Input: part model. Units: mm. Frame: model coordinates. Face numbers are marked on the shaded views. A direction names the side the tool comes from. Give positions to 0.01 mm unless a question says otherwise; leave off trailing zeros. Write each loop counter-clockwise with the first axis right and the second up, starting at its lowest first coordinate (ties: lowest second). Pieces come first, ordered by that corner, then holes. Notation, with made-up numbers: (46.25, 78.25) -> (50.25, 78.25) arc R22 cw to (50.25, 107.25) -> close; hole circle Ø9 at (6, 55.5). An arc over 180 degrees is marked (long way). Return JSON: item names as keys, results as strings. Group by question number.
Item 1: Section B-B, the plane z = 5. Return loops of the section in (x, y).
Item 2: Pin query (flat end, axial travel): P1, Ø0.7, axis at y = 4, z = -4.5, coming from the +X side; P2, Ø6, axis at x = 20.5, y = 5, coming from the -Z side; P3, Ø10, axis at x = 19, y = 15, coming from the -Z side; P4, Ø4, axis at x = 35.5, z = -8, coming from the -Y side. Return the tip coordinate at first contact, or that it passes through.
Item 3: Section D-D, the plane x = 20. Return loops of the section in (y, z), then the cut area to 3 significant figures.
Item 4: Mould query, pull axis Y, two halves, no side actions, for the marked faces 4, 5, 6 and 7. Classes: released by +Y, released by -Y, zero draft, split by the parting line, or undercut.
Item 5: Set-up query: the marked faces 1, 2 and 3. Return all of +Z, -Z, +X, -X, +Y, -Y with unobstructed straight access to the full face (end or side cutting, diameter ignored); none if empty.
Item 6: Section A-A, the plane y = 13.5. Return loops of the section in (x, z), then the cut area to 3 significant figures.
Item 7: Line query: line 1 (X direction, y = 17.5, z = 8); line 2 (Y direction, x = 29, z = 15); line 3 (X direction, y = 2.05, z = 25.2). Output: solid intervals per line, ascending. Write a range as [from, to].
Item 8: Section C-C, the plane x = 14. Return loops of the section in (y, z).
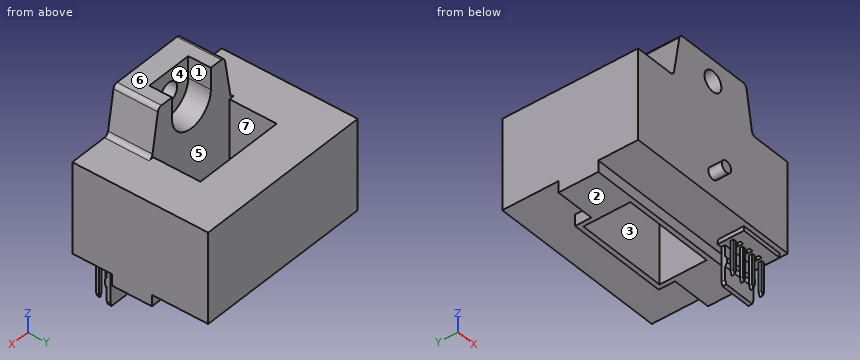
from build123d import *

# Parameters (mm, degrees)
SKETCH1_W                   = 40
SKETCH1_H                   = 30
SKETCH1_W_2                 = 20.4
SKETCH1_H_2                 = 10.4
BOSS_EXTRUDE1_DEPTH         = 20
BOSS_EXTRUDE2_DEPTH         = 9.8
CUT_EXTRUDE1_DEPTH          = 5
SKETCH4_R                   = 2.25
CUT_EXTRUDE2_DEPTH          = 56.991427915
SKETCH5_W                   = 8.8
SKETCH5_H                   = 8.8
SKETCH5_W_2                 = 20.4
SKETCH5_H_2                 = 10.4
BOSS_EXTRUDE3_DEPTH         = 2.5
SKETCH7_R                   = 1.25
BOSS_EXTRUDE4_DEPTH         = 3
BODY_MOVE_COPY6_START       = 1
BODY_MOVE_COPY6_DEPTH       = 4.9
BODY_MOVE_COPY6_START_2     = 5.95
BODY_MOVE_COPY6_2_DEPTH     = 0.85
BODY_MOVE_COPY6_START_3     = 3.8825
BODY_MOVE_COPY6_3_DEPTH     = 0.635
BODY_MOVE_COPY6_4_OUTLINE_W = 0.75
BODY_MOVE_COPY6_4_OUTLINE_H = 1
BODY_MOVE_COPY6_4_DEPTH     = 2.35
BODY_MOVE_COPY6_START_4     = 4.6
BODY_MOVE_COPY6_5_OUTLINE_W = 0.75
BODY_MOVE_COPY6_5_OUTLINE_H = 1
BODY_MOVE_COPY6_5_DEPTH     = 1.35
BODY_MOVE_COPY6_START_5     = 30.5
BODY_MOVE_COPY6_6_DEPTH     = 7.5
BODY_MOVE_COPY6_START_6     = 29.5
BODY_MOVE_COPY6_7_DEPTH     = 9.5


with BuildPart() as part:
    # Sketch1 → Boss-Extrude1 (new body)
    with BuildSketch(Plane.XY):
        with Locations((20, 15)):
            Rectangle(SKETCH1_W, SKETCH1_H)
        with Locations((20, 15)):
            Rectangle(SKETCH1_W_2, SKETCH1_H_2, mode=Mode.SUBTRACT)
    extrude(amount=BOSS_EXTRUDE1_DEPTH)

    # Sketch2 → Boss-Extrude2 (add)
    with BuildSketch(Plane.XZ):
        with BuildLine():
            Line((8.6, 20), (31.4, 20))
            ThreePointArc((31.4, 20), (30.755366169, 20.23550851), (30.414365834, 20.831105526))
            Line((30.414365834, 20.831105526), (28.985634166, 29.168894474))
            ThreePointArc((28.985634166, 29.168894474), (28.644633831, 29.76449149), (28, 30))
            Line((28, 30), (12, 30))
            ThreePointArc((12, 30), (11.355366169, 29.76449149), (11.014365834, 29.168894474))
            Line((11.014365834, 29.168894474), (9.585634166, 20.831105526))
            ThreePointArc((9.585634166, 20.831105526), (9.244633831, 20.23550851), (8.6, 20))
        make_face()
    extrude(amount=-BOSS_EXTRUDE2_DEPTH)

    # Sketch3 → Cut-Extrude1 (cut)
    with BuildSketch(Plane(origin=(0, 9.8, 0), x_dir=(1, 0, 0), z_dir=(0, 1, 0))):
        with BuildLine():
            Line((25.2, -25.2), (25.2, -30))
            Line((25.2, -30), (14.8, -30))
            Line((14.8, -30), (14.8, -25.2))
            ThreePointArc((14.8, -25.2), (20, -20), (25.2, -25.2))
        make_face()
    extrude(amount=-CUT_EXTRUDE1_DEPTH, mode=Mode.SUBTRACT)

    # Sketch4 → Cut-Extrude2 (cut, through all)
    with BuildSketch(Plane(origin=(0, 4.8, 0), x_dir=(1, 0, 0), z_dir=(0, 1, 0))):
        with Locations(Location((20, -25.2, 0), (0, 0, 270))):
            Circle(SKETCH4_R)
    extrude(amount=-CUT_EXTRUDE2_DEPTH, mode=Mode.SUBTRACT)

    # Sketch5 → Boss-Extrude3 (add)
    # profile 1 of 3: a face of its own
    with BuildSketch(Plane(origin=(0, 0, 0), x_dir=(-1, 0, 0), z_dir=(0, 0, -1))):
        with Locations((-4.4, 13.2)):
            Rectangle(SKETCH5_W, SKETCH5_H)
    # profile 2 of 3: a face of its own
    with BuildSketch(Plane(origin=(0, 0, 0), x_dir=(-1, 0, 0), z_dir=(0, 0, -1))):
        Polygon((-31.2, 8.8), (-8.8, 8.8), (-8.8, 17.6), (-8.8, 21.2), (-31.2, 21.2), (-31.2, 17.6), align=None)
        with Locations((-20, 15)):
            Rectangle(SKETCH5_W_2, SKETCH5_H_2, mode=Mode.SUBTRACT)
    # profile 3 of 3: a face of its own
    with BuildSketch(Plane(origin=(0, 0, 0), x_dir=(-1, 0, 0), z_dir=(0, 0, -1))):
        with Locations((-35.6, 13.2)):
            Rectangle(SKETCH5_W, SKETCH5_H)
    extrude(amount=BOSS_EXTRUDE3_DEPTH)

    # Sketch7 → Boss-Extrude4 (add)
    with BuildSketch(Plane.XZ):
        with Locations(Location((20, 5, 0), (0, 0, 90))):
            Circle(SKETCH7_R)
    extrude(amount=BOSS_EXTRUDE4_DEPTH)


with BuildPart() as body_2:
    # Body-Move/Copy6: read off the stored shape, not the designer's step
    # Body-Move/Copy6 outline → Body-Move/Copy6 (new body)
    with BuildSketch(Plane(origin=(0, 0, 0), x_dir=(1, 0, 0), z_dir=(0, 1, 0)).offset(BODY_MOVE_COPY6_START)):
        Polygon((34.75, -1.3), (36.25, -1.3), (36.25, -2.3), (37.25, -2.3), (37.25, -1.3), (38.75, -1.3), (38.75, -2.3), (39, -2.3), (39, 1), (37.125, 1), (37.125, 0), (36.375, 0), (36.375, 1), (34.625, 1), (34.625, 0), (33.875, 0), (33.875, 1), (32.125, 1), (32.125, 0), (31.375, 0), (31.375, 1), (29.5, 1), (29.5, -2.3), (29.75, -2.3), (29.75, -1.3), (31.25, -1.3), (31.25, -2.3), (32.25, -2.3), (32.25, -1.3), (33.75, -1.3), (33.75, -2.3), (34.75, -2.3), align=None)
    extrude(amount=BODY_MOVE_COPY6_DEPTH)

    # Body-Move_Copy6 2 outline → Body-Move_Copy6 2 (add)
    with BuildSketch(Plane(origin=(0, 0, 0), x_dir=(1, 0, 0), z_dir=(0, 1, 0)).offset(BODY_MOVE_COPY6_START_2)):
        Polygon((38, 1), (38, 8.6), (37.708823813, 9.4), (30.791176187, 9.4), (30.5, 8.6), (30.5, 1), align=None)
    extrude(amount=BODY_MOVE_COPY6_2_DEPTH)

    # Body-Move_Copy6 3 outline → Body-Move_Copy6 3 (add)
    with BuildSketch(Plane(origin=(0, 0, 0), x_dir=(1, 0, 0), z_dir=(0, 1, 0)).offset(BODY_MOVE_COPY6_START_3)):
        Polygon((35.1825, -4.827675919), (35.5, -5.7), (35.8175, -4.827675919), (35.8175, -1.3), (35.1825, -1.3), align=None)
        Polygon((38.3175, -1.3), (37.6825, -1.3), (37.6825, -4.827675919), (38, -5.7), (38.3175, -4.827675919), align=None)
        Polygon((33.3175, -4.827675919), (33.3175, -1.3), (32.6825, -1.3), (32.6825, -4.827675919), (33, -5.7), align=None)
        Polygon((38.3175, 1), (38.3175, 7.627675919), (38, 8.5), (37.6825, 7.627675919), (37.6825, 1), align=None)
        Polygon((30.8175, -4.827675919), (30.8175, -1.3), (30.1825, -1.3), (30.1825, -4.827675919), (30.5, -5.7), align=None)
        Polygon((35.1825, 1), (35.8175, 1), (35.8175, 7.627675919), (35.5, 8.5), (35.1825, 7.627675919), align=None)
        Polygon((30.1825, 7.627675919), (30.1825, 1), (30.8175, 1), (30.8175, 7.627675919), (30.5, 8.5), align=None)
        Polygon((32.6825, 1), (33.3175, 1), (33.3175, 7.627675919), (33, 8.5), (32.6825, 7.627675919), align=None)
    extrude(amount=BODY_MOVE_COPY6_3_DEPTH)

    # Body-Move_Copy6 4 outline → Body-Move_Copy6 4 (add)
    with BuildSketch(Plane(origin=(0, 0, 0), x_dir=(1, 0, 0), z_dir=(0, 1, 0)).offset(BODY_MOVE_COPY6_START)):
        with Locations((36.75, 0.5)):
            Rectangle(BODY_MOVE_COPY6_4_OUTLINE_W, BODY_MOVE_COPY6_4_OUTLINE_H)
        with Locations((34.25, 0.5)):
            Rectangle(BODY_MOVE_COPY6_4_OUTLINE_W, BODY_MOVE_COPY6_4_OUTLINE_H)
        with Locations((31.75, 0.5)):
            Rectangle(BODY_MOVE_COPY6_4_OUTLINE_W, BODY_MOVE_COPY6_4_OUTLINE_H)
    extrude(amount=BODY_MOVE_COPY6_4_DEPTH)

    # Body-Move_Copy6 5 outline → Body-Move_Copy6 5 (add)
    with BuildSketch(Plane(origin=(0, 0, 0), x_dir=(1, 0, 0), z_dir=(0, 1, 0)).offset(BODY_MOVE_COPY6_START_4)):
        with Locations((36.75, 0.5)):
            Rectangle(BODY_MOVE_COPY6_5_OUTLINE_W, BODY_MOVE_COPY6_5_OUTLINE_H)
        with Locations((34.25, 0.5)):
            Rectangle(BODY_MOVE_COPY6_5_OUTLINE_W, BODY_MOVE_COPY6_5_OUTLINE_H)
        with Locations((31.75, 0.5)):
            Rectangle(BODY_MOVE_COPY6_5_OUTLINE_W, BODY_MOVE_COPY6_5_OUTLINE_H)
    extrude(amount=BODY_MOVE_COPY6_5_DEPTH)

    # Body-Move_Copy6 6 outline → Body-Move_Copy6 6 (add)
    with BuildSketch(Plane.YZ.offset(BODY_MOVE_COPY6_START_5)):
        Polygon((5.95, -3.5), (5.55, -3.976701437), (5.55, -4.976701437), (5.95, -5.66952176), align=None)
        with BuildLine():
            Line((5.9, -1), (6.8, -1))
            Line((6.8, -1), (6.8, -0.6))
            ThreePointArc((6.8, -0.6), (6.536396103, 0.036396103), (5.9, 0.3))
            Line((5.9, 0.3), (5.9, -1))
        make_face()
    extrude(amount=BODY_MOVE_COPY6_6_DEPTH)

    # Body-Move_Copy6 7 outline → Body-Move_Copy6 7 (add)
    with BuildSketch(Plane.YZ.offset(BODY_MOVE_COPY6_START_6)):
        with BuildLine():
            Line((5.9, -1), (6.8, -1))
            Line((6.8, -1), (6.8, -0.6))
            ThreePointArc((6.8, -0.6), (6.536396103, 0.036396103), (5.9, 0.3))
            Line((5.9, 0.3), (5.9, -1))
        make_face()
    extrude(amount=BODY_MOVE_COPY6_7_DEPTH)


with BuildPart() as part_1:
    add(part.part)

    # Intersect3: read off the stored shape, not the designer's step
    # Intersect3: union body 2
    add(body_2.part)


solid = part_1.part
Answer below:
{
 "1": {"outline": "(0, 0) -> (18.75, 0) -> (18.75, -3) -> (21.25, -3) -> (21.25, 0) -> (40, 0) -> (40, 30) -> (0, 30) -> close; hole (9.8, 9.8) -> (30.2, 9.8) -> (30.2, 20.2) -> (9.8, 20.2) -> close"},
 "2": {"P1": "stops at x = 38.32", "P2": "stops at z = 0", "P3": "passes through", "P4": "stops at y = 3.88"},
 "3": {"outline": "(-3, 3.75) -> (0, 3.75) -> (0, 0) -> (8.8, 0) -> (8.8, -2.5) -> (9.8, -2.5) -> (9.8, 20) -> (4.8, 20) -> (4.8, 22.95) -> (0, 22.95) -> (0, 6.25) -> (-3, 6.25) -> close; (0, 27.45) -> (4.8, 27.45) -> (4.8, 30) -> (0, 30) -> close; (20.2, -2.5) -> (21.2, -2.5) -> (21.2, 0) -> (30, 0) -> (30, 20) -> (20.2, 20) -> close", "area": "431 mm2"},
 "4": {"face 4": "released by +Y", "face 5": "undercut", "face 6": "zero draft", "face 7": "undercut"},
 "5": {"face 1": "+Z, +Y", "face 2": "-Z, +X, -X, +Y", "face 3": "+Z, -Z"},
 "6": {"outline": "(0, -2.5) -> (9.8, -2.5) -> (9.8, 20) -> (0, 20) -> close; (30.2, -2.5) -> (40, -2.5) -> (40, 20) -> (30.2, 20) -> close", "area": "441 mm2"},
 "7": {"line 1": "x = [0, 9.8], [30.2, 40]", "line 2": "y = [0, 9.8], [20.2, 30]", "line 3": "x = [10.33, 17.75], [22.25, 29.67]"},
 "8": {"outline": "(0, 0) -> (8.8, 0) -> (8.8, -2.5) -> (9.8, -2.5) -> (9.8, 30) -> (0, 30) -> close; (20.2, -2.5) -> (21.2, -2.5) -> (21.2, 0) -> (30, 0) -> (30, 20) -> (20.2, 20) -> close"}
}
